The listing builds one solid part. Answer for the finished solid, in the listing's coordinates (mm). Face numbers are marked on the shaded views. A direction names the side the tool comes from. Coordinates: 2 decimals unless noted, no trailing zeros. Order: outer loops, then holes, each group sorted by start corner. A loop starts at its lowest first (then second) coordinate and runs counter-clockwise, first axis right, second up. Notation, with made-up numbers: (35.25, 10.25) -> (63.25, 10.25) arc R11 cw to (63.25, 30.25) -> close; hole circle Ø5 at (59.25, -26.5). An arc over 180 degrees is marked (long way). Answer in a Markdown table with one row per item.
```python
from build123d import *

# Parameters (mm, degrees)
SKETCH1_W           = 12.7
SKETCH1_H           = 12.7
BOSS_EXTRUDE1_DEPTH = 2.54
FILLET1_R           = 0.635
SHELL1_START        = 0.635
SHELL1_OUTLINE_W    = 1.905
SHELL1_OUTLINE_H    = 11.43
SHELL1_DEPTH        = 11.43
SKETCH2_R           = 2.54
BOSS_EXTRUDE2_DEPTH = 1.905
BOSS_EXTRUDE3_DEPTH = 0.00254


# Read off the part's stored shape, not the designer's step: Shell1
with BuildPart() as part:
    # Sketch1 → Boss-Extrude1 (new body)
    with BuildSketch(Plane(origin=(0, 0, 0), x_dir=(1, 0, 0), z_dir=(0, 1, 0))):
        with Locations((6.35, 6.35)):
            Rectangle(SKETCH1_W, SKETCH1_H)
    extrude(amount=BOSS_EXTRUDE1_DEPTH)

    # Fillet1
    fillet1_edges = [part.edges().sort_by_distance(p)[0] for p in [
        (0, 1.27, -12.7),
        (12.7, 1.27, -12.7),
        (12.7, 1.27, 0),
        (0, 1.27, 0),
    ]]
    fillet(fillet1_edges, radius=FILLET1_R)

    # Shell1 outline → Shell1 (cut)
    with BuildSketch(Plane.YZ.offset(SHELL1_START)):
        with Locations((0.9525, -6.35)):
            Rectangle(SHELL1_OUTLINE_W, SHELL1_OUTLINE_H)
    extrude(amount=SHELL1_DEPTH, mode=Mode.SUBTRACT)

    # Sketch2 → Boss-Extrude2 (add)
    with BuildSketch(Plane(origin=(0, 1.905, 0), x_dir=(-1, 0, 0), z_dir=(0, -1, 0))):
        with Locations(Location((-6.35, 6.35, 0), (0, 0, 270))):
            Circle(SKETCH2_R)
    extrude(amount=BOSS_EXTRUDE2_DEPTH)

    # Sketch3 → Boss-Extrude3 (add)
    with BuildSketch(Plane(origin=(0, 2.54, 0), x_dir=(1, 0, 0), z_dir=(0, 1, 0))):
        Polygon((6.411642829, 5.27375641), (6.931269231, 4.418948718), (6.50513742, 4.418948718), (5.710115385, 5.27375641), align=None)
        with BuildLine():
            Line((5.080325641, 8.333153846), (5.080325641, 8.903025641))
            add(Edge.make_bspline(
                [(5.080325641, 8.903025641), (5.107116622, 8.919158467), (5.158856938, 8.950315128), (5.235918867, 8.991651266), (5.309205163, 9.027027273), (5.379088546, 9.055681099), (5.445318097, 9.07824066), (5.507802803, 9.094263611), (5.566750704, 9.104549048), (5.605002578, 9.105899018), (5.623484696, 9.106551282)],
                knots=[0, 0, 0, 0, 1.279207482, 2.470480605, 3.576080812, 4.606860037, 5.558565817, 6.435744397, 7.244200283, 8, 8, 8, 8], degree=3))
            add(Edge.make_bspline(
                [(5.623484696, 9.106551282), (5.647252633, 9.10608216), (5.696197248, 9.10511611), (5.770940929, 9.096225937), (5.849121635, 9.082896049), (5.932404463, 9.063232193), (6.024309741, 9.035772523), (6.128219217, 8.999075098), (6.245748934, 8.952611932), (6.327892985, 8.91646479), (6.371441426, 8.897301482)],
                knots=[0, 0, 0, 0, 0.728864224, 1.500928647, 2.306032779, 3.161048191, 4.124103712, 5.247132966, 6.540575143, 8, 8, 8, 8], degree=3))
            add(Edge.make_bspline(
                [(6.371441426, 8.897301482), (6.398937756, 8.884854189), (6.448424397, 8.862452119), (6.515501601, 8.834429807), (6.566641046, 8.814091133), (6.596124718, 8.804955011), (6.608039984, 8.801262821)],
                knots=[0, 0, 0, 0, 1.417318505, 2.550825291, 3.414343566, 4, 4, 4, 4], degree=3))
            add(Edge.make_bspline(
                [(6.608039984, 8.801262821), (6.633154743, 8.795327171), (6.682531311, 8.783657459), (6.733229124, 8.781815384), (6.758140144, 8.780910256)],
                knots=[0, 0, 0, 0, 1.01727437, 2, 2, 2, 2], degree=3))
            add(Edge.make_bspline(
                [(6.758140144, 8.780910256), (6.778737764, 8.781558102), (6.820988878, 8.782887003), (6.885281854, 8.792925647), (6.951980152, 8.809139744), (7.021102843, 8.831372247), (7.092577195, 8.860369751), (7.166290369, 8.895358707), (7.242337948, 8.937076476), (7.292957038, 8.968303502), (7.319107692, 8.984435897)],
                knots=[0, 0, 0, 0, 0.817691354, 1.677299118, 2.577777856, 3.541554841, 4.557701377, 5.638471298, 6.779995431, 8, 8, 8, 8], degree=3))
            Line((7.319107692, 8.984435897), (7.319107692, 8.414564103))
            add(Edge.make_bspline(
                [(7.319107692, 8.414564103), (7.296635434, 8.398350673), (7.252631937, 8.366602748), (7.184346346, 8.325219904), (7.116456359, 8.290374664), (7.049081778, 8.261073651), (6.981942418, 8.239048359), (6.915204166, 8.222851078), (6.848756076, 8.21290154), (6.804390317, 8.211657593), (6.782308814, 8.211038462)],
                knots=[0, 0, 0, 0, 1.138472114, 2.229270987, 3.277482784, 4.272796559, 5.24538971, 6.177327133, 7.09282843, 8, 8, 8, 8], degree=3))
            add(Edge.make_bspline(
                [(6.782308814, 8.211038462), (6.734070736, 8.212764993), (6.636621448, 8.216252887), (6.527110127, 8.237556451), (6.451666575, 8.258503219), (6.406550833, 8.271812301), (6.356134507, 8.289361286), (6.29953379, 8.308711319), (6.237551107, 8.332007692), (6.169954271, 8.357956857), (6.096218469, 8.386587733), (6.04555015, 8.407472659), (6.01908766, 8.418380208)],
                knots=[0, 0, 0, 0, 1.816478987, 3.669602728, 4.183070076, 4.766772394, 5.441136484, 6.19386005, 7.020227999, 7.935420581, 8.921734247, 10, 10, 10, 10], degree=3))
            add(Edge.make_bspline(
                [(6.01908766, 8.418380208), (6.002332613, 8.424935618), (5.970509168, 8.437386536), (5.925038155, 8.455476927), (5.883685286, 8.471352947), (5.846629194, 8.48526161), (5.813753702, 8.496906564), (5.785288756, 8.506272562), (5.761265135, 8.514230216), (5.723286502, 8.52375686), (5.669365237, 8.534055878), (5.621424075, 8.535803844), (5.597407973, 8.536679487)],
                knots=[0, 0, 0, 0, 1.224273616, 2.325305503, 3.329974039, 4.238366513, 5.01858254, 5.702877263, 6.277757238, 6.739620974, 8.366714654, 10, 10, 10, 10], degree=3))
            add(Edge.make_bspline(
                [(5.597407973, 8.536679487), (5.579145964, 8.536202288), (5.542464937, 8.535243786), (5.487640677, 8.527022953), (5.432392514, 8.515183006), (5.375489546, 8.496720769), (5.313776653, 8.469947593), (5.24415197, 8.43419635), (5.164904001, 8.387896903), (5.109853792, 8.352265842), (5.080325641, 8.333153846)],
                knots=[0, 0, 0, 0, 0.776252433, 1.559178841, 2.353291584, 3.177347174, 4.098437677, 5.211375113, 6.504221197, 8, 8, 8, 8], degree=3))
        make_face()
    extrude(amount=BOSS_EXTRUDE3_DEPTH)


solid = part.part
```
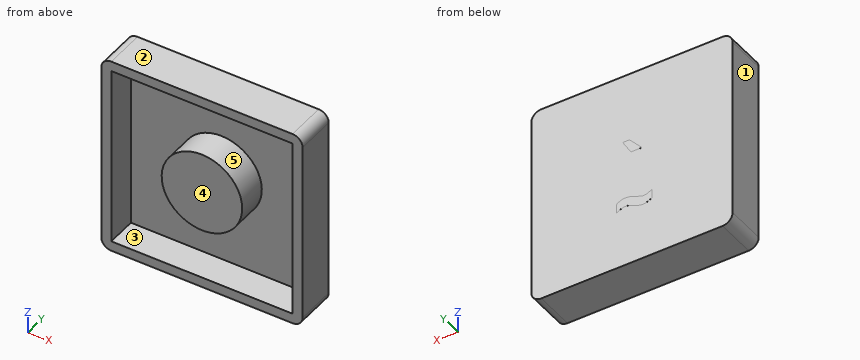
(1) A cutting plane is placed at A-A, the plane y = 1.4. Determine the outline of the cut face in (x, z) (3 decimals).
Check values:
| item | result |
|---|---|
| outline | (0, -12.065) arc R0.635 ccw to (0.635, -12.7) -> (12.065, -12.7) arc R0.635 ccw to (12.7, -12.065) -> (12.7, -0.635) arc R0.635 ccw to (12.065, 0) -> (0.635, 0) arc R0.635 ccw to (0, -0.635) -> close; circle Ø5.08 at (6.35, -6.35); hole (0.635, -12.065) -> (12.065, -12.065) -> (12.065, -0.635) -> (0.635, -0.635) -> close |
(2) A cutting plane is placed at D-D, the plane x = 7.75. Determine the outline of the cut face in (y, z) (3 decimals).
Check values:
| item | result |
|---|---|
| outline | (0, -12.7) -> (2.54, -12.7) -> (2.54, 0) -> (0, 0) -> (0, -0.635) -> (1.905, -0.635) -> (1.905, -4.231) -> (0, -4.231) -> (0, -8.469) -> (1.905, -8.469) -> (1.905, -12.065) -> (0, -12.065) -> close |
(3) Which of the six approach directions +Z, -Z, +X, -X, +Y, -Y give full straight-line access (tool end or side, diameter ignored) to the marked faces 4 and 5?
Check values:
| item | result |
|---|---|
| face 4 | +Z, -Z, +X, -X, -Y |
| face 5 | -Y |
(4) Find the intervals of material crossed by line 1 along Z through (x, y) = (9.25, 0.7) (3 decimals); line 2 along X through (y, z) = (0.2, -0.75) (3 decimals); line 3 along Z through (x, y) = (4.75, 1.75) (3 decimals), in increasing order. Write a range as from..to.
Check values:
| item | result |
|---|---|
| line 1 | -12.7..-12.065, -0.635..0 |
| line 2 | 0..0.635, 12.065..12.7 |
| line 3 | -12.7..-12.065, -8.323..-4.377, -0.635..0 |
(5) For a pull along X with two mould halves and no side action, classify the marked faces 1, 2 and 3 as released by +X, released by -X, zero draft, split by the parting line, or undercut.
Check values:
| item | result |
|---|---|
| face 1 | released by -X |
| face 2 | zero draft |
| face 3 | undercut |
(6) A cutting plane is placed at C-C, the plane x = 10.75. Determine the outline of the cut face in (y, z) (3 decimals).
Check values:
| item | result |
|---|---|
| outline | (0, -12.7) -> (2.54, -12.7) -> (2.54, 0) -> (0, 0) -> (0, -0.635) -> (1.905, -0.635) -> (1.905, -12.065) -> (0, -12.065) -> close |
(7) A cutting plane is placed at B-B, the plane z = -6.35. Determine the outline of the cut face in (x, y) (3 decimals), then the cut area to 3 significant figures.
Check values:
| item | result |
|---|---|
| outline | (0, 0) -> (0.635, 0) -> (0.635, 1.905) -> (3.81, 1.905) -> (3.81, 0) -> (8.89, 0) -> (8.89, 1.905) -> (12.065, 1.905) -> (12.065, 0) -> (12.7, 0) -> (12.7, 2.54) -> (0, 2.54) -> close |
| area | 20.2 mm² |
